Geometry: see drawing. Coordinates: mm, zero at the bounding-box minimum. Coordinates: 2 decimals unless noted, no trailing zeros. Loops run counter-clockwise (first coordinate to the right, second up) from the corner with the lowest first, then second, coordinate; pieces in that order, holes last. Notation, with made-up numbers: (77.25, 77.25) - (95.25, 77.25) arc R17 cw to (95.25, 95.25) - close; hole circle Ø3 at (36.25, -15.5). An arc over 180 degrees is marked (long way). Answer in a Markdown table with one row per item.
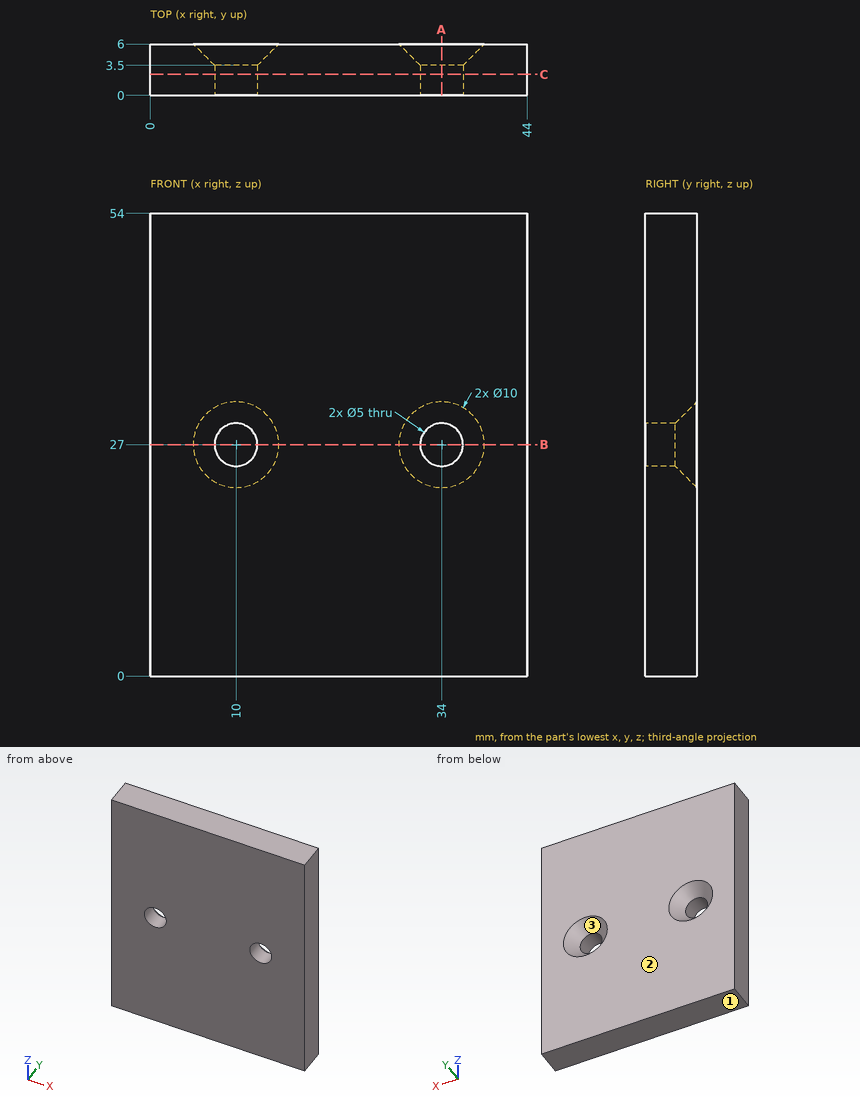
(1) Ray query, probe 1 along X at (y, z) = (2.3, 27); probe 2 along Z at (x, y) = (10, 1.3); probe 3 along Z at (x, y) = (10.5, 3.3). Return the intervals inside material, ascending.
Verdict:
| item | result |
|---|---|
| probe 1 | x = 0 to 7.5, 12.5 to 31.5, 36.5 to 44 |
| probe 2 | z = 0 to 24.5, 29.5 to 54 |
| probe 3 | z = 0 to 24.55, 29.45 to 54 |
(2) Cut plane A-A on x = 34. Output: boundary loops of the cut face in (y, z), then the cut area to 3 significant figures.
Verdict:
| item | result |
|---|---|
| outline | (0, 0) - (6, 0) - (6, 22) - (3.5, 24.5) - (0, 24.5) - close; (0, 29.5) - (3.5, 29.5) - (6, 32) - (6, 54) - (0, 54) - close |
| area | 288 mm² |
(3) Pull-direction query (Z, two-part tool) for the marked faces 1, 2 and 3; classes: pulls with the +Z half, pulls with the -Z half, needs draft (parallel to the pull), parting line crosses it, or undercut.
Verdict:
| item | result |
|---|---|
| face 1 | pulls with the -Z half |
| face 2 | needs draft |
| face 3 | undercut |
(4) Cut plane B-B on z = 27. Output: boundary loops of the cut face in (x, y), then the cut area to 4 significant figures.
Verdict:
| item | result |
|---|---|
| outline | (0, 0) - (7.5, 0) - (7.5, 3.5) - (5, 6) - (0, 6) - close; (12.5, 0) - (31.5, 0) - (31.5, 3.5) - (29, 6) - (15, 6) - (12.5, 3.5) - close; (36.5, 0) - (44, 0) - (44, 6) - (39, 6) - (36.5, 3.5) - close |
| area | 191.5 mm² |
(5) First-contact query: pin 1 Ø3 at (x, y) = (12, 2.5) entering from -Z. Flat tip, straight axial feed; report the tip coordinate or a pass-through.
Verdict:
| item | result |
|---|---|
| pin 1 | stops at z = 0 |
(6) Cut plane C-C on y = 2.45. Output: boundary loops of the cut face in (x, z), then the cut area to 3 significant figures.
Verdict:
| item | result |
|---|---|
| outline | (0, 0) - (44, 0) - (44, 54) - (0, 54) - close; hole circle Ø5 at (10, 27); hole circle Ø5 at (34, 27) |
| area | 2,340 mm² |
